Can you work these out from the model? Positions are in its coordinate system, mm. A direction names the side the tool comes from. Give positions to 0.01 mm unless a question says otherwise; leave off trailing zeros. Order: outer loops, then holes, each group sorted by start corner. A loop starts at its lowest first (then second) coordinate and runs counter-clockwise, first axis right, second up. Notation, with made-up numbers: M 64.5,4.25 L 93.5,4.25 A28 cw 93.5,37.25 Z; hole C 26.5,-18.5 d8. An arc over 180 degrees is marked long. Use a Markdown table: item, result. Add a question column.
from build123d import *

# Parameters (mm, degrees)
F0_W     = 10
F0_H     = 120
F0_W_2   = 31.2
F0_H_2   = 18
F1_DEPTH = 2
F3_W     = 2
F3_H     = 18
F3_W_2   = 18
F3_H_2   = 2
F4_DEPTH = 7
F5_R     = 4.99999


# Not quite as in the source:
# - a fillet or chamfer is up to 0.001 mm smaller than in the source, because OpenCascade refuses the exact size


with BuildPart() as f1:
    # F0 (on Top) → F1 (new body)
    with BuildSketch(Plane.XY):
        Polygon((9, 135.3739356415), (-9, 135.3739356415), (-9, 76.6739356415), (-9, 58.6739356415), (-9, -18.0260643585), (9, -18.0260643585), (9, 58.6739356415), (9, 76.6739356415), align=None)
        with Locations((0, 51.9739356415)):
            Rectangle(F0_W, F0_H, mode=Mode.SUBTRACT)
        with Locations((-24.6, 67.6739356415)):
            Rectangle(F0_W_2, F0_H_2)
        with Locations((24.6, 67.6739356415)):
            Rectangle(F0_W_2, F0_H_2)
    extrude(amount=F1_DEPTH)

    # F3 (on face) → F4 (join)
    with BuildSketch(Plane.XY.offset(2)):
        with Locations((-39.2, 67.6739356415)):
            Rectangle(F3_W, F3_H)
        with Locations((39.2, 67.6739356415)):
            Rectangle(F3_W, F3_H)
        with Locations((0, 134.3739356415)):
            Rectangle(F3_W_2, F3_H_2)
        with Locations((0, -17.0260643585)):
            Rectangle(F3_W_2, F3_H_2)
    extrude(amount=F4_DEPTH)

    # F5 (radius 5 in the source; OpenCascade refuses exactly that, so slightly less here)
    f5_edges = [f1.edges().sort_by_distance(p)[0] for p in [
        (-9, 58.673936, 1),
        (9, 58.673936, 1),
        (9, 76.673936, 1),
        (-9, 76.673936, 1),
        (-5, 111.973936, 1),
        (5, 111.973936, 1),
    ]]
    fillet(f5_edges, radius=F5_R)


solid = f1.part
1. I need wall thicknesses on L1, parallel to Y at x = -5, z = 6.75; L2, parallel to X at y = 85.5, z = 1; L3, parallel to Y at x = -35, z = 1.5. Which ranges of each line are inside material? Lowest first, please. Write a range as [from, to].
2. If we section it at C-C, the plane x = -7.5: List the corners of the cut face in (y, z) for me.
3. If we section it at B-B, the plane y = 105: List the corners of the cut face in (x, z) for me.
4. On a 3-axis mill with a long thin cutter (end or side, diameter ignored), from which of +Z, -Z, +X, -X, +Y, -Y can I reach the whole of each face in a straight line? I mean faces 4 (the face through (9, 12.3, 1.8)), 5 (the face through (-30.1, 58.674, 1.8)), 6 (the face through (-38.2, 68, 5)). Say none if no direction works.
5. We'd pull the mould along Y, two halves only. Please class faces 1 (the face through (0, -16.026, 5)), 2 (the face through (29, 76.674, 1)), 3 (the face through (40.2, 68, 4)): +Y half, -Y half, draft (parallel to the pull), parting line (faces both ways), or undercut.
6. If we section it at D-D, the plane x = -31.5: List the corners of the cut face in (y, z) for me.
7. Will these pins go through, and if not, where does the flat tip stop? pin 1 (4.5 mm diameter, centred on x = -26.5, z = 5, fed in from -Y); pin 2 (10 mm diameter, centred on x = 17, y = 65.5, fed in from +Z); pin 3 (1 mm diameter, centred on y = 44.5, z = 1.5, fed in from -X); pin 4 (4.5 mm diameter, centred on y = 109.5, z = 4, fed in from +X).
8. If we section it at A-A, the plane z = 6: List the corners of the cut face in (x, y) for me, then the cut area to 3 significant figures.
Geometry results:
| question | item | result |
|---|---|---|
| 1 | L1 | y = [-18.03, -16.03], [133.37, 135.37] |
| 1 | L2 | x = [-9, -5], [5, 9] |
| 1 | L3 | y = [58.67, 76.67] |
| 2 | outline | M -18.03,0 L 135.37,0 L 135.37,9 L 133.37,9 L 133.37,2 L -16.03,2 L -16.03,9 L -18.03,9 Z |
| 3 | outline | M -9,0 L -5,0 L -5,2 L -9,2 Z; M 5,0 L 9,0 L 9,2 L 5,2 Z |
| 4 | face 4 | +Z, -Z, +X, -Y |
| 4 | face 5 | +Z, -Z, -X, -Y |
| 4 | face 6 | +Z, +Y, -Y |
| 5 | face 1 | undercut |
| 5 | face 2 | +Y half |
| 5 | face 3 | draft |
| 6 | outline | M 58.67,0 L 76.67,0 L 76.67,2 L 58.67,2 Z |
| 7 | pin 1 | passes through |
| 7 | pin 2 | stops at z = 2 |
| 7 | pin 3 | stops at x = -9 |
| 7 | pin 4 | stops at x = 9 |
| 8 | outline | M -40.2,58.67 L -38.2,58.67 L -38.2,76.67 L -40.2,76.67 Z; M -9,-18.03 L 9,-18.03 L 9,-16.03 L -9,-16.03 Z; M -9,133.37 L 9,133.37 L 9,135.37 L -9,135.37 Z; M 38.2,58.67 L 40.2,58.67 L 40.2,76.67 L 38.2,76.67 Z |
| 8 | area | 144 mm^2 |
